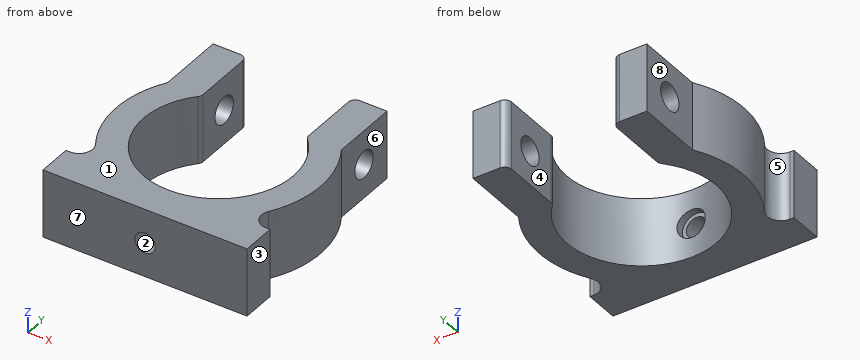
Autodesk Inventor part; units mm, degrees
ref_plane "YZ Plane" through (0, 0, 0) normal (1, 0, 0) x (0, 1, 0)
ref_plane "XZ Plane" through (0, 0, 0) normal (0, 1, 0) x (-1, 0, 0)
ref_plane "XY Plane" through (0, 0, 0) normal (0, 0, 1) x (1, 0, 0)
sketch "Sketch1" plane through (0, 0, 0) normal (0, 0, 1) x (1, 0, 0)
  arc A0 (-7.7782, 7.7782) -> (7.7782, 7.7782) centre (0, 0) ccw
  line L0 (7.7782, 7.7782) -> (11.0228, 11.0228)
  line L1 (0, 0) -> (15.5887, 0) construction
  line L2 (0, 0) -> (20, 0) construction
  line L3 (-7.7782, 7.7782) -> (-10.6066, 10.6066)
  line L4 (15, -11) -> (15, -16)
  line L5 (15, -16) -> (-15, -16)
  line L6 (-15, -16) -> (-15, -11)
  line L7 (-15, -11) -> (-10.198, -11)
  arc A1 (-10.6066, 10.6066) -> (-10.198, -11) centre (0, 0) ccw
  arc A2 (10.198, -11) -> (10.6066, 10.6066) centre (0, 0) ccw
  line L8 (15, -11) -> (10.198, -11)
  dimension "d6" = 5
  dimension "d7" = 30
extrude "Extrusion1" add sketch "Sketch1" along normal blind 10
sketch "Sketch2" plane through (-15, -16, 0) normal (0, -1, 0) x (1, 0, 0)
  line L0 (0, 10) -> (30, 10)
  line L1 (30, 10) -> (25.198, 10)
  line L2 (0, 0) -> (30, 0)
  circle A0 centre (15, 5) radius 1.5
  point P0 (15, 0)
  dimension "d10" = 3
extrude "Extrusion2" cut sketch "Sketch2" against normal blind 24.75
sketch "Sketch3" plane through (10.198, -11, 0) normal (0, 1, 0) x (1, 0, 0)
  line L0 (4.802, 0) -> (0, 0)
  line L1 (-20.3961, -10) -> (-25.198, -10)
  line L2 (-20.3961, 0) -> (-25.198, 0)
  line L3 (4.802, -10) -> (0, -10)
  circle A0 centre (-10.198, -5) radius 2.0833
  point P0 (-10.198, 0)
sketch "Sketch4" plane through (0, 0, 0) normal (0, 0, -1) x (-1, 0, 0)
  point P0 (0, 0)
extrude "Extrusion3" cut sketch "Sketch3" against normal blind 1
sketch "Sketch5" plane through (10.198, -11, 0) normal (0, -1, 0) x (1, 0, 0)
  arc A0 (-10.198, 3.5) -> (-10.198, 6.5) centre (-10.198, 5) ccw
  arc A1 (-10.198, 2.9167) -> (-10.198, 7.0833) centre (-10.198, 5) ccw
  circle A2 centre (-10.198, 5) radius 2.0833
  point P0 (-10.198, 0)
  point P1 (-10.198, 2.9167)
extrude "Extrusion4" cut sketch "Sketch5" against normal blind 1.5
fillet "Fillet1" radius 2 1 edges at (-10.198, -11, 5)
fillet "Fillet2" radius 2 1 edges at (10.198, -11, 5)
sketch "Sketch6" plane through (0, 0, 10) normal (0, 0, 1) x (1, 0, 0)
  line L0 (-7.7782, 7.7782) -> (-10.6066, 10.6066)
  line L1 (-7.7782, 7.7782) -> (-7.7782, 17.7782)
  line L2 (-7.7782, 17.7782) -> (-12.7782, 17.7782)
  line L3 (-12.7782, 17.7782) -> (-12.7782, 7.8561)
  arc A0 (-10.6066, 10.6066) -> (-12.7255, -7.9412) centre (0, 0) ccw
  dimension "d21" = 10
  dimension "d22" = 5
extrude "Extrusion5" add sketch "Sketch6" against normal blind 10
sketch "Sketch7" plane through (0, 0, 10) normal (0, 0, 1) x (1, 0, 0)
  line L0 (7.7782, 7.7782) -> (7.7782, 17.7782)
  line L1 (7.7782, 17.7782) -> (12.7782, 17.7782)
  line L2 (12.7782, 17.7782) -> (12.7782, 7.8561)
  arc A0 (12.7255, -7.9412) -> (10.6066, 10.6066) centre (0, 0) ccw
  arc A1 (-7.7782, 7.7782) -> (7.7782, 7.7782) centre (0, 0) ccw
  line L3 (7.7782, 7.7782) -> (12.7782, 7.8561)
  dimension "d25" = 5
extrude "Extrusion6" add sketch "Sketch7" against normal blind 10
sketch "Sketch8" plane through (12.7782, 7.8561, 10) normal (1, 0, 0) x (0, 0, -1)
  line L0 (0, 9.9221) -> (0, 0) construction
  line L1 (10, -0.0779) -> (0, -0.0779) construction
  line L2 (0, 9.9221) -> (10, -0.0779) construction
  line L3 (0, 9.9221) -> (10, 9.9221) construction
  line L4 (10, 9.9221) -> (0, -0.0779) construction
  circle A0 centre (5, 4.9221) radius 2
  point P0 (10, -7.8561)
  dimension "d28" = 4
extrude "Extrusion7" cut sketch "Sketch8" against normal blind 36
fillet "Fillet5" radius 1 1 edges at (-7.7782, 17.7782, 5)
fillet "Fillet6" radius 1 1 edges at (-7.7782, 7.7782, 5)
fillet "Fillet7" radius 1 1 edges at (7.7782, 17.7782, 5)
fillet "Fillet8" radius 1 1 edges at (7.7782, 7.7782, 5)
properties part number "buisClip"
Geometry: final body of the model. Coordinates: model frame, mm. Face numbers are marked on the shaded views. A direction names the side the tool comes from. Round coordinates to 2 decimals unless told otherwise and drop trailing zeros. Order: outer loops, then holes, each group sorted by start corner. A loop starts at its lowest first (then second) coordinate and runs counter-clockwise, first axis right, second up. Notation, with made-up numbers: (56.5, 0.25) -> (78.5, 0.25) arc R34 ccw to (78.5, 30.25) -> close; hole circle Ø6 at (16, -36). An arc over 180 degrees is marked (long way). Use one line per item in the form item = value.
(1) Section B-B on x = 0.5. Return loops of the section in (y, z).
Results list:
outline = (-16, 0) -> (-10.99, 0) -> (-10.99, 2.98) -> (-12, 2.98) -> (-12, 3.59) -> (-16, 3.59) -> close; (-16, 6.41) -> (-12, 6.41) -> (-12, 7.02) -> (-10.99, 7.02) -> (-10.99, 10) -> (-16, 10) -> close
(2) Section A-A on y = 0. Return loops of the section in (x, z).
Results list:
outline = (-15, 0) -> (-11, 0) -> (-11, 10) -> (-15, 10) -> close; (11, 0) -> (15, 0) -> (15, 10) -> (11, 10) -> close
(3) Section D-D on z = 9. Return loops of the section in (x, y).
Results list:
outline = (-15, -16) -> (15, -16) -> (15, -11) -> (14.42, -11) arc R2 cw to (12.73, -7.94) arc R15 ccw to (12.78, 7.86) -> (12.78, 17.78) -> (8.78, 17.78) arc R1 ccw to (7.78, 16.78) -> (7.78, 8.18) arc R1 ccw to (8.05, 7.5) arc R11 cw (long way) to (-8.05, 7.5) arc R1 ccw to (-7.78, 8.18) -> (-7.78, 16.78) arc R1 ccw to (-8.78, 17.78) -> (-12.78, 17.78) -> (-12.78, 7.86) arc R15 ccw to (-12.73, -7.94) arc R2 cw to (-14.42, -11) -> (-15, -11) -> close
(4) Ray query, probe 1 along Y at (x, z) = (-8.5, 4.5); probe 2 along Y at (x, z) = (-9.75, 5); probe 3 along X at (y, z) = (15, 5.5). Return the intervals inside material, ascending. Write a range as [from, to].
Results list:
probe_1 = [-16, -6.98], [6.98, 10.84], [14.71, 17.74]
probe_2 = [-16, -5.09], [5.09, 10.78], [14.78, 17.78]
probe_3 = [-12.78, -7.78], [7.78, 12.78]
(5) First-contact query: pin 1 Ø3 at (y, z) = (12.78, 5) entering from -X; pin 2 Ø2 at (x, z) = (0, 6) entering from +Y; pin 3 Ø2 at (x, z) = (-7.5, 1.5) entering from +Y; pin 4 Ø3 at (y, z) = (11.5, 5) entering from +X. Flat tips, straight axial feed; report the tip coordinate or a pass-through.
Results list:
pin_1 = through
pin_2 = -12
pin_3 = 17.74
pin_4 = 12.78
(6) Access query for the marked faces 4, 5, 6, 7 and 8. Directions: +Z, -Z, +X, -X, +Y, -Y. A direction counts if a zero-diameter tool reaches every point of the face in a straight line with its end or side. Return the directions, or none.
Results list:
face_4 = +Z, -Z, +Y
face_5 = +Z, -Z, -X
face_6 = +Z, -Z, +X, +Y
face_7 = +Z, -Z, +X, -X, -Y
face_8 = +Z, -Z, -X, +Y
(7) Draft query along Z for the marked faces 1, 2 and 3. Return one class per face: pulls with the +Z half, pulls with the -Z half, needs draft (parallel to the pull), parting line crosses it, or undercut.
Results list:
face_1 = pulls with the +Z half
face_2 = undercut
face_3 = needs draft
(8) Section C-C on y = -14. Return loops of the section in (x, z).
Results list:
outline = (-15, 0) -> (15, 0) -> (15, 10) -> (-15, 10) -> close; hole circle Ø3 at (0, 5)
